from build123d import *

# Parameters (mm, degrees)
SKETCH_1_R          = 2
EXTRUDE_1_DEPTH     = 52
SKETCH_2_R          = 4
EXTRUDE_2_DEPTH     = 4
CUT_EXTRUDE_1_DEPTH = 2


with BuildPart() as part:
    # 草图1 → 凸台-拉伸1 (new body)
    with BuildSketch(Plane.XY):
        with Locations(Location((0, 0, 0), (0, 0, 180))):
            Circle(SKETCH_1_R)
    extrude(amount=EXTRUDE_1_DEPTH)

    # 草图2 → 凸台-拉伸2 (add)
    with BuildSketch(Plane(origin=(0, 0, 0), x_dir=(-1, 0, 0), z_dir=(0, 0, -1))):
        Circle(SKETCH_2_R)
    extrude(amount=EXTRUDE_2_DEPTH)

    # 草图3 → 切除-拉伸1 (cut)
    with BuildSketch(Plane(origin=(0, 0, -4), x_dir=(-1, 0, 0), z_dir=(0, 0, -1))):
        Polygon((2, 0), (1, 1.732050808), (-1, 1.732050808), (-2, 0), (-1, -1.732050808), (1, -1.732050808), align=None)
    extrude(amount=-CUT_EXTRUDE_1_DEPTH, mode=Mode.SUBTRACT)


solid = part.part
For this review, take the finished solid that the model builds, in its own axes (mm). A direction names the side the tool comes from. Coordinates: 2 decimals unless noted, no trailing zeros. Loops run counter-clockwise (first coordinate to the right, second up) from the corner with the lowest first, then second, coordinate; pieces in that order, holes last. Notation, with made-up numbers: (-5, 63.5) -> (27, 63.5) arc R19 cw to (27, 95.5) -> close; hole circle Ø1 at (-27.5, -17.75). An arc over 180 degrees is marked (long way). Write each question's results on one line, items separated by ' | '.
Q1. Add section B-B, the plane z = 23.5. State the section outline as (x, y) points.
Taken from the geometry:
outline: circle Ø4 at (0, 0)
Q2. Mouldability with a two-part tool opening along X and no side actions: class faces 1 (the cylindrical face through (0.867, -3.905, -1.972)), 2 (the flat face through (0, 2, -4)), 3 (the flat face through (-1.49, -0.88, -3.01)) as +X half, -X half, draft (parallel to the pull), parting line (faces both ways), or undercut.
Taken from the geometry:
face 1: parting line | face 2: draft | face 3: undercut
Q3. Add section C-C, the plane y = 1. State the section outline as (x, z) points.
Taken from the geometry:
outline: (-3.87, -4) -> (-1.42, -4) -> (-1.42, -2) -> (1.42, -2) -> (1.42, -4) -> (3.87, -4) -> (3.87, 0) -> (1.73, 0) -> (1.73, 52) -> (-1.73, 52) -> (-1.73, 0) -> (-3.87, 0) -> close
Q4. For pin 1 Ø3 at (x, z) = (-1.5, 42.5) entering from -Y; pin 2 Ø2 at (x, y) = (-1, 3) entering from +Z; pin 3 Ø4 at (y, z) = (-0.5, 12.5) entering from -X, all flat-tipped, find the tip position at first contact; note any pin that passes through.
Taken from the geometry:
pin 1: y = -2 | pin 2: z = 0 | pin 3: x = -2
Q5. To check wall thickness, follow line 1 along Z through (x, y) = (-1, 3.75); line 2 along X through (y, z) = (1, 43.5); line 3 along Z through (x, y) = (1.5, -0.5). State the ranges of each line that lie inside material, in increasing order. Write a range as [from, to].
Taken from the geometry:
line 1: [-4, 0] | line 2: [-1.73, 1.73] | line 3: [-2, 52]
Q6. Add section D-D, the plane x = -2.5. State the section outline as (y, z) points.
Taken from the geometry:
outline: (-3.12, -4) -> (3.12, -4) -> (3.12, 0) -> (-3.12, 0) -> close
Q7. Add section A-A, the plane x = 0. State the section outline as (y, z) points, then the cut area to 3 significant figures.
Taken from the geometry:
outline: (-4, -4) -> (-1.73, -4) -> (-1.73, -2) -> (1.73, -2) -> (1.73, -4) -> (4, -4) -> (4, 0) -> (2, 0) -> (2, 52) -> (-2, 52) -> (-2, 0) -> (-4, 0) -> close | area: 233 mm²
Q8. Machinability: for faces 4 (the cylindrical face through (0, 2, 26)), 5 (the flat face through (0, -1.732, -3)), 6 (the flat face through (0, 0, 52)), which of the approach directions +Z, -Z, +X, -X, +Y, -Y give a long, thin tool a straight path to every point of the face, cutting with its end or side? Answer none if there is none.
Taken from the geometry:
face 4: +Z | face 5: -Z | face 6: +Z, +X, -X, +Y, -Y
